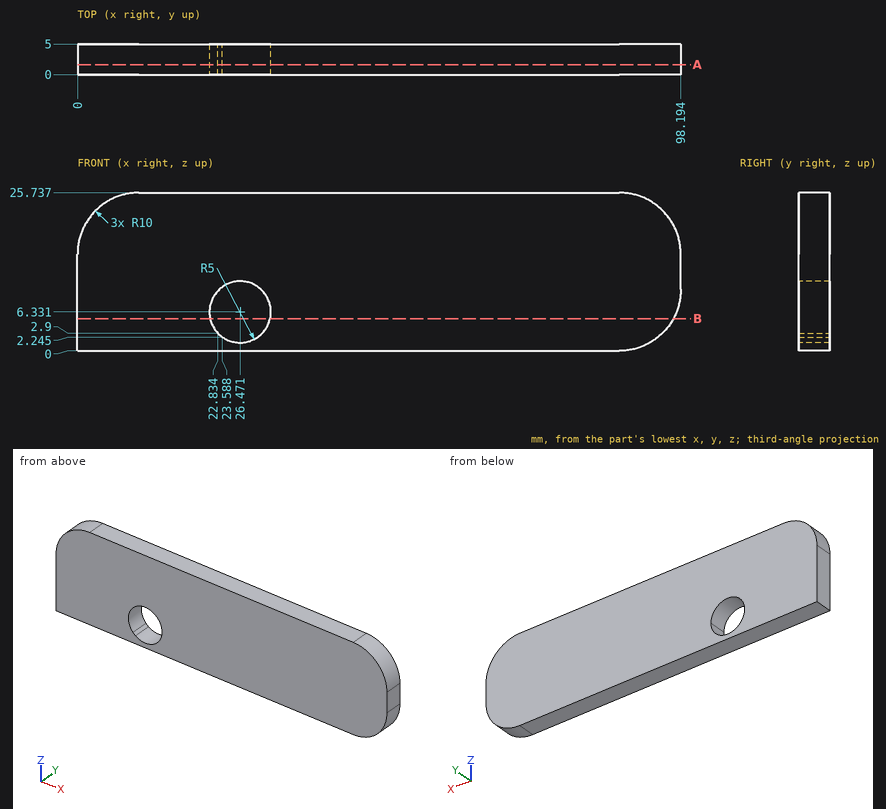
Answer from the drawing. Dimensions are ordinates in mm from the lowest x, y and z of the part. Coordinates: 2 decimals unless noted, no trailing zeros. Order: outer loops, then holes, each group sorted by start corner. A loop starts at its lowest first (then second) coordinate and runs counter-clockwise, first axis right, second up. Notation, with made-up numbers: (22, 81.5) - (27, 81.5) arc R19 cw to (27, 87.5) - close; hole circle Ø9 at (19.25, -29). An arc over 180 degrees is marked (long way). Answer as a JSON object with one key per item and string values. Group by question number.
Item 1: Consider probe 1 along X at (y, z) = (2.7, 6.5) (1 decimal); probe 2 along X at (y, z) = (1.8, 16.25); probe 3 along X at (y, z) = (3.95, 7.5). Determine where each line is inside the solid, lowest interval first. Write a range as from..to.
Item 2: Section A-A (y = 1.65) is taken. Give the vertices of the cut face in (x, z) (1 decimal).
Item 3: Section B-B (z = 5.25) is taken. Give the vertices of the cut face in (x, y), plus the area to 3 significant figures.
Results are:
{
 "1": {"probe 1": "x = 0..21.5, 31.5..97.6", "probe 2": "x = 0.01..98.18", "probe 3": "x = 0..21.61, 31.33..97.88"},
 "2": {"outline": "(0, 0) - (88.2, 0) arc R10 ccw to (98.2, 10) - (98.2, 15.7) arc R10 ccw to (88.2, 25.7) - (10, 25.7) arc R10 ccw to (0, 15.7) - close; hole (22.8, 2.9) - (23.6, 2.2) arc R5 ccw to (31.5, 6.3) arc R5 ccw to (23.4, 10.3) arc R5 ccw to start"},
 "3": {"outline": "(0, 0) - (21.59, 0) - (21.59, 5) - (0, 5) - close; (31.35, 0) - (96.99, 0) - (96.99, 5) - (31.35, 5) - close", "area": "436 mm^2"}
}
